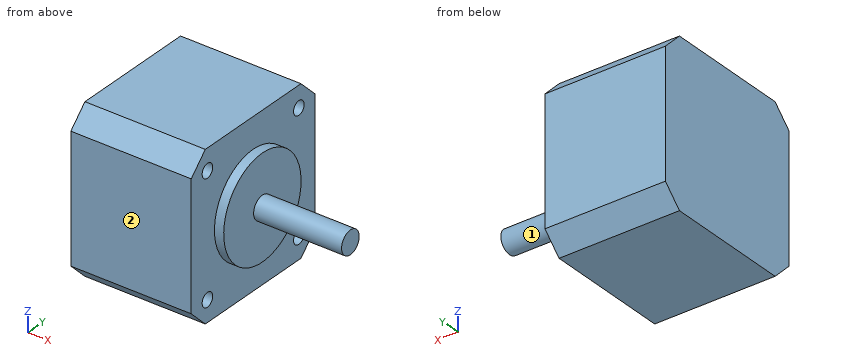
from build123d import *

# Parameters (mm, degrees)
SKETCH1_R           = 2.5
BOSS_EXTRUDE1_DEPTH = 19
SKETCH2_R           = 11
BOSS_EXTRUDE2_DEPTH = 2
SKETCH3_W           = 35.2
SKETCH3_H           = 35.2
SKETCH3_R           = 1.5
BOSS_EXTRUDE3_DEPTH = 4
SKETCH4_W           = 35.2
SKETCH4_H           = 35.2
BOSS_EXTRUDE4_DEPTH = 22
CHAMFER1_SIZE       = 4


with BuildPart() as part:
    # Sketch1 → Boss-Extrude1 (new body)
    with BuildSketch(Plane(origin=(0, 0, 0), x_dir=(0, 0, -1), z_dir=(1, 0, 0))):
        Circle(SKETCH1_R)
    extrude(amount=-BOSS_EXTRUDE1_DEPTH)

    # Sketch2 → Boss-Extrude2 (add)
    with BuildSketch(Plane.ZY.offset(19)):
        Circle(SKETCH2_R)
    extrude(amount=BOSS_EXTRUDE2_DEPTH)

    # Sketch3 → Boss-Extrude3 (add)
    with BuildSketch(Plane.ZY.offset(21)):
        Rectangle(SKETCH3_W, SKETCH3_H)
        with Locations((-13, 13)):
            Circle(SKETCH3_R, mode=Mode.SUBTRACT)
        with Locations((13, 13)):
            Circle(SKETCH3_R, mode=Mode.SUBTRACT)
        with Locations((13, -13)):
            Circle(SKETCH3_R, mode=Mode.SUBTRACT)
        with Locations((-13, -13)):
            Circle(SKETCH3_R, mode=Mode.SUBTRACT)
    extrude(amount=BOSS_EXTRUDE3_DEPTH)

    # Sketch4 → Boss-Extrude4 (add)
    with BuildSketch(Plane.ZY.offset(25)):
        Rectangle(SKETCH4_W, SKETCH4_H)
    extrude(amount=BOSS_EXTRUDE4_DEPTH)

    # Chamfer1
    chamfer1_edges = [part.edges().sort_by_distance(p)[0] for p in [
        (-34, -17.6, 17.6),
        (-34, 17.6, 17.6),
        (-34, 17.6, -17.6),
        (-34, -17.6, -17.6),
    ]]
    chamfer(chamfer1_edges, length=CHAMFER1_SIZE)


solid = part.part
Model file for the job. Use its own axes, mm. Face numbers are marked on the shaded views. A direction names the side the tool comes from. Coordinates: 2 decimals unless noted, no trailing zeros. Order: outer loops, then holes, each group sorted by start corner. A loop starts at its lowest first (then second) coordinate and runs counter-clockwise, first axis right, second up. Notation, with made-up numbers: (89, 77) -> (126, 77) arc R30 cw to (126, 110) -> close; hole circle Ø8 at (41.5, 0). An arc over 180 degrees is marked (long way). Return JSON: item names as keys, results as strings. Group by question number.
Item 1: Saw through at D-D on x = -7. Write the cut outline in (y, z).
Item 2: Wall check: line 1 along Y through (x, z) = (-22.6, 13); line 2 along X through (y, z) = (1, -3.5); line 3 along X through (y, z) = (-2, 11). Give the ranges that are in metal, low to high. Write a range as [from, to].
Item 3: Tool access for the marked faces 1 and 2: list every direction of +Z, -Z, +X, -X, +Y, -Y with a clear straight run to the whole face (end or side of a thin tool).
Item 4: Saw through at A-A on z = 13. Write the cut outline in (x, y).
Item 5: Flat gauge pins, fed straight in: P1, Ø3.5, axis at y = -13, z = 13, coming from the +X side; P2, Ø0.9, axis at y = 13, z = 12.5, coming from the +X side. Where does each tip first touch, or does it go through?
Item 6: Saw through at B-B on x = -23.5. Write the cut outline in (y, z), then the cut area to 3 significant figures.
Values found:
{
 "1": {"outline": "circle Ø5 at (0, 0)"},
 "2": {"line 1": "y = [-17.6, -14.5], [-11.5, 11.5], [14.5, 17.6]", "line 2": "x = [-47, -19]", "line 3": "x = [-47, -21]"},
 "3": {"face 1": "+X", "face 2": "+Z, -Z, +X, -X, -Y"},
 "4": {"outline": "(-47, -17.6) -> (-21, -17.6) -> (-21, -14.5) -> (-25, -14.5) -> (-25, -11.5) -> (-21, -11.5) -> (-21, 11.5) -> (-25, 11.5) -> (-25, 14.5) -> (-21, 14.5) -> (-21, 17.6) -> (-47, 17.6) -> close"},
 "5": {"P1": "stops at x = -21", "P2": "stops at x = -25"},
 "6": {"outline": "(-17.6, -13.6) -> (-13.6, -17.6) -> (13.6, -17.6) -> (17.6, -13.6) -> (17.6, 13.6) -> (13.6, 17.6) -> (-13.6, 17.6) -> (-17.6, 13.6) -> close; hole circle Ø3 at (-13, -13); hole circle Ø3 at (-13, 13); hole circle Ø3 at (13, -13); hole circle Ø3 at (13, 13)", "area": "1,180 mm2"}
}
